```python
from build123d import *

# Parameters (mm, degrees)
F0_R      = 28.575
F0_R_2    = 2.032
F1_DEPTH  = 3.175
F2_R      = 13.97
F3_DEPTH  = 6.35
F4_R      = 12.0015
F5_DEPTH  = 22.225
F7_DEPTH  = 31.75
F9_R      = 1.4224
F10_DEPTH = 0.3175
F11_R     = 2.794
F12_DEPTH = 3.81


with BuildPart() as f1:
    # F0 (on Top) → F1 (new body)
    with BuildSketch(Plane.XY):
        Circle(F0_R)
        with Locations((-20.6222299276, -11.90625)):
            Circle(F0_R_2, mode=Mode.SUBTRACT)
        with Locations((0, -23.8125)):
            Circle(F0_R_2, mode=Mode.SUBTRACT)
        with Locations((20.6222299276, -11.90625)):
            Circle(F0_R_2, mode=Mode.SUBTRACT)
        with Locations((-20.6222299276, 11.90625)):
            Circle(F0_R_2, mode=Mode.SUBTRACT)
        with Locations((20.6222299276, 11.90625)):
            Circle(F0_R_2, mode=Mode.SUBTRACT)
        with Locations((0, 23.8125)):
            Circle(F0_R_2, mode=Mode.SUBTRACT)
    extrude(amount=F1_DEPTH)

    # F2 (on face) → F3 (join)
    with BuildSketch(Plane.XY.offset(3.175)):
        Circle(F2_R)
    extrude(amount=F3_DEPTH)

    # F4 (on face) → F5 (join)
    with BuildSketch(Plane.XY.offset(9.525)):
        Circle(F4_R)
    extrude(amount=F5_DEPTH)

    # F6 (on face) → F7 (cut, through all)
    with BuildSketch(Plane(origin=(0, 0, 0), x_dir=(1, 0, 0), z_dir=(0, 0, -1))):
        with BuildLine():
            ThreePointArc((-2.0635057548, 2.413), (-1.3283437485, -2.8837697352), (3.175, 0))
            ThreePointArc((3.175, 0), (2.8837697352, 1.3283437485), (2.0635057548, 2.413))
            Line((2.0635057548, 2.413), (0, 2.413))
            Line((0, 2.413), (-2.0635057548, 2.413))
        make_face()
    extrude(amount=-F7_DEPTH, mode=Mode.SUBTRACT)

    # F9 (on offset) → F10 (cut, through all)
    with BuildSketch(Plane.XZ.offset(14.2875)):
        with Locations((0, 6.35)):
            Circle(F9_R)
    extrude(amount=-F10_DEPTH, mode=Mode.SUBTRACT)

    # F11 (on offset) → F12 (cut)
    with BuildSketch(Plane.XZ.offset(14.2875)):
        with Locations((0, 6.35)):
            Circle(F11_R)
    extrude(amount=-F12_DEPTH, mode=Mode.SUBTRACT)


solid = f1.part
```
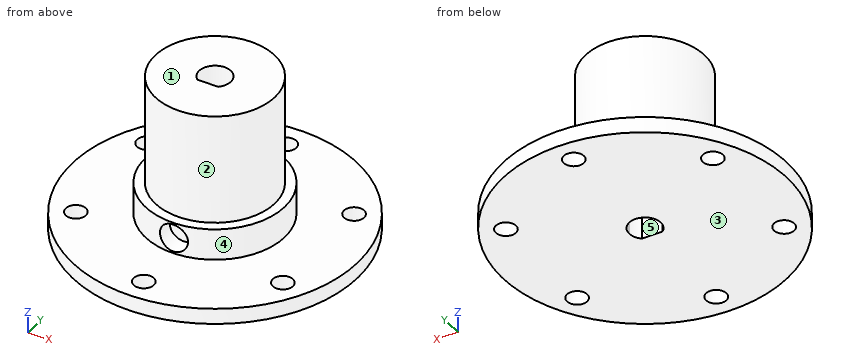
Source: CAD feature listing. Evaluate the final solid. Frame: model axes, mm. Face numbers are marked on the shaded views. A direction names the side the tool comes from. Give positions to 0.01 mm unless a question says otherwise; leave off trailing zeros. Loops run counter-clockwise (first coordinate to the right, second up) from the corner with the lowest first, then second, coordinate; pieces in that order, holes last. Notation, with made-up numbers: (55.5, -27) -> (97.5, -27) arc R34 cw to (97.5, 7) -> close; hole circle Ø4 at (-10.75, 24). An arc over 180 degrees is marked (long way). Use a Markdown table: item, result. Add a question column.
(1) Pull-direction query (X, two-part tool) for the marked faces 3, 4 and 5; classes: +X half, -X half, draft (parallel to the pull), parting line (faces both ways), or undercut.
(2) First-contact query: pin 1 Ø3 at (y, z) = (9.5, 18) entering from +X; pin 2 Ø3.5 at (x, z) = (0, 18.5) entering from +Y; pin 3 Ø5.5 at (x, y) = (-20.62, 11.91) entering from +Z (3 decimals). Flat tips, straight axial feed; report the tip coordinate or a pass-through.
(3) Access query for the marked faces 1 and 2. Directions: +Z, -Z, +X, -X, +Y, -Y. A direction counts if a zero-diameter tool reaches every point of the face in a straight line with its end or side. Return the directions, or none.
(4) Section query C-C (y = -23). Output: boundary loops of the cut face in (x, z) (3 decimals), then the cut area to 3 significant figures.
(5) Ray query, line 1 (Y direction, x = 0, z = 1) (1 decimal); line 2 (Z direction, x = -7.5, y = -14) (3 decimals); line 3 (Y direction, x = 0, z = 24) (1 decimal). Return the intervals inside material, ascending.
(6) Section query A-A (x = 0). Count the separate pieces of the cut face and the enclosed holes in it, then the cut area to 3 significant figures.
Checked values:
| question | item | result |
|---|---|---|
| 1 | face 3 | draft |
| 1 | face 4 | parting line |
| 1 | face 5 | undercut |
| 2 | pin 1 | x = 8.95 |
| 2 | pin 2 | y = 12 |
| 2 | pin 3 | z = 3.175 |
| 3 | face 1 | +Z, +X, -X, +Y, -Y |
| 3 | face 2 | +Z |
| 4 | outline | (-16.957, 0) -> (-1.862, 0) -> (-1.862, 3.175) -> (-16.957, 3.175) -> close; (1.862, 0) -> (16.957, 0) -> (16.957, 3.175) -> (1.862, 3.175) -> close |
| 4 | area | 95.8 mm^2 |
| 5 | line 1 | -28.6 to -25.8, -21.8 to -2.4, 3.2 to 21.8, 25.8 to 28.6 |
| 5 | line 2 | 0 to 3.175 |
| 5 | line 3 | -12 to -2.4, 3.2 to 12 |
| 6 | separate pieces | 4 |
| 6 | enclosed holes | 0 |
| 6 | area | 670 mm^2 |
